The listing builds one solid part. Answer for the finished solid, in the listing's coordinates (mm). A direction names the side the tool comes from. Give positions to 0.01 mm unless a question says otherwise; leave off trailing zeros. Order: outer loops, then holes, each group sorted by start corner. A loop starts at its lowest first (then second) coordinate and runs counter-clockwise, first axis right, second up. Notation, with made-up numbers: (4, -3) - (42, -3) arc R13 ccw to (42, 19) - close; hole circle Ø1 at (86, -24). An arc over 180 degrees is marked (long way). Answer in a Markdown table with one row per item.
from build123d import *

# Parameters (mm, degrees)
SKETCH1_R                     = 9.5
SKETCH1_W                     = 7
SKETCH1_H                     = 1.9
BOSS_EXTRUDE1_DEPTH           = 50
SKETCH32_W                    = 32.172664372
SKETCH32_H                    = 50
SKETCH32_W_2                  = 30.763378825
BOSS_EXTRUDE4_DEPTH           = 3
SKETCH30_R                    = 1.675
SKETCH30_R_2                  = 1.25
CUT_EXTRUDE14_DEPTH           = 84.200435696
SKETCH31_R                    = 4
CUT_EXTRUDE15_DEPTH           = 2
CHAMFER1_SIZE                 = 1
SKETCH36_R                    = 2
CUT_EXTRUDE18_DEPTH           = 83.371475645
SKETCH37_R                    = 4
CUT_EXTRUDE19_DEPTH           = 2.8
SKETCH38_W                    = 7.194206864
SKETCH38_H                    = 7.080700956
BOSS_EXTRUDE6_DEPTH           = 6
BOSS_EXTRUDE6_DRAFT           = 20
BOSS_EXTRUDE6_PROFILE_2_DEPTH = 6
BOSS_EXTRUDE6_PROFILE_2_DRAFT = 20
FILLET2_R                     = 2
CHAMFER2_SIZE                 = 0.5
CUT_EXTRUDE20_START           = -10
SKETCH39_W                    = 33.713665857
SKETCH39_H                    = 35.884460507
CUT_EXTRUDE20_DEPTH           = 67.252868798
CUT_EXTRUDE21_DEPTH           = 83.371475645
CUT_EXTRUDE21_DEPTH_BACK      = 83.371475645
CHAMFER3_SIZE                 = 1
FILLET3_R                     = 2


with BuildPart() as part:
    # Sketch1 → Boss-Extrude1 (new body)
    with BuildSketch(Plane.XY):
        with BuildLine():
            Line((-34.408656248, 2.4), (34.408656248, 2.4))
            ThreePointArc((34.408656248, 2.4), (36.148562201, 2.95608362), (37.243446021, 4.418181818))
            ThreePointArc((37.243446021, 4.418181818), (52.24014746, 13.312841145), (63.5, 0))
            ThreePointArc((63.5, 0), (59.545941546, -9.545941546), (50, -13.5))
            ThreePointArc((50, -13.5), (42.170423209, -10.99762371), (37.243446021, -4.418181818))
            ThreePointArc((37.243446021, -4.418181818), (36.148562201, -2.95608362), (34.408656248, -2.4))
            Line((34.408656248, -2.4), (12.372954376, -2.4))
            ThreePointArc((12.372954376, -2.4), (10.729786704, -2.89001992), (9.623408959, -4.2))
            ThreePointArc((9.623408959, -4.2), (0, -10.5), (-9.623408959, -4.2))
            ThreePointArc((-9.623408959, -4.2), (-10.729786704, -2.89001992), (-12.372954376, -2.4))
            Line((-12.372954376, -2.4), (-34.408656248, -2.4))
            ThreePointArc((-34.408656248, -2.4), (-36.148562201, -2.95608362), (-37.243446021, -4.418181818))
            ThreePointArc((-37.243446021, -4.418181818), (-42.170423209, -10.99762371), (-50, -13.5))
            ThreePointArc((-50, -13.5), (-59.545941546, -9.545941546), (-63.5, 0))
            ThreePointArc((-63.5, 0), (-52.24014746, 13.312841145), (-37.243446021, 4.418181818))
            ThreePointArc((-37.243446021, 4.418181818), (-36.148562201, 2.95608362), (-34.408656248, 2.4))
        make_face()
        with Locations((50, 0)):
            Circle(SKETCH1_R, mode=Mode.SUBTRACT)
        with Locations(Location((-50, 0, 0), (0, 0, 180))):
            Circle(SKETCH1_R, mode=Mode.SUBTRACT)
        with Locations((0, -7.2)):
            Rectangle(SKETCH1_W, SKETCH1_H, mode=Mode.SUBTRACT)
    extrude(amount=BOSS_EXTRUDE1_DEPTH)

    # Sketch32 → Boss-Extrude4 (add)
    with BuildSketch(Plane.XZ.offset(2.4)):
        with Locations((-22.574766715, 25)):
            Rectangle(SKETCH32_W, SKETCH32_H)
        with Locations((23.370404996, 25)):
            Rectangle(SKETCH32_W_2, SKETCH32_H)
    extrude(amount=BOSS_EXTRUDE4_DEPTH)

    # Sketch30 → Cut-Extrude14 (cut, through all)
    with BuildSketch(Plane(origin=(0, -6.25, 0), x_dir=(1, 0, 0), z_dir=(0, 1, 0))):
        with Locations(Location((-0.160776584, -5, 0), (0, 0, 90))):
            Circle(SKETCH30_R)
        with Locations(Location((-0.160776584, -20, 0), (0, 0, 90))):
            Circle(SKETCH30_R)
        with Locations(Location((14.839223416, -12.5, 0), (0, 0, 90))):
            Circle(SKETCH30_R_2)
        with Locations(Location((-15.160776584, -12.5, 0), (0, 0, 90))):
            Circle(SKETCH30_R_2)
    extrude(amount=CUT_EXTRUDE14_DEPTH, mode=Mode.SUBTRACT)

    # Sketch31 → Cut-Extrude15 (cut)
    with BuildSketch(Plane(origin=(0, 2.4, 0), x_dir=(1, 0, 0), z_dir=(0, 1, 0))):
        with Locations(Location((-0.160776584, -5, 0), (0, 0, 270))):
            Circle(SKETCH31_R)
        with Locations(Location((-0.160776584, -20, 0), (0, 0, 270))):
            Circle(SKETCH31_R)
    extrude(amount=-CUT_EXTRUDE15_DEPTH, mode=Mode.SUBTRACT)

    # Chamfer1
    chamfer1_edges = [part.edges().sort_by_distance(p)[0] for p in [
        (0, -6.25, 0),
        (0, -6.25, 50),
    ]]
    chamfer(chamfer1_edges, length=CHAMFER1_SIZE)

    # Sketch36 → Cut-Extrude18 (cut, through all)
    with BuildSketch(Plane(origin=(0, 2.4, 0), x_dir=(1, 0, 0), z_dir=(0, 1, 0))):
        with Locations(Location((30, -10, 0), (0, 0, 270))):
            Circle(SKETCH36_R)
        with Locations(Location((-30, -10, 0), (0, 0, 270))):
            Circle(SKETCH36_R)
    extrude(amount=-CUT_EXTRUDE18_DEPTH, mode=Mode.SUBTRACT)

    # Sketch37 → Cut-Extrude19 (cut)
    with BuildSketch(Plane.XZ.offset(5.4)):
        with Locations((30, 10)):
            Circle(SKETCH37_R)
        with Locations((-30, 10)):
            Circle(SKETCH37_R)
    extrude(amount=-CUT_EXTRUDE19_DEPTH, mode=Mode.SUBTRACT)


with BuildPart() as boss_extrude6_tool:
    # Sketch38 → Boss-Extrude6 (with draft: the straight prism first)
    with BuildSketch(Plane(origin=(0, 2.4, 0), x_dir=(1, 0, 0), z_dir=(0, 0, 1))):
        with Locations((18.597103432, 0)):
            Rectangle(SKETCH38_W, SKETCH38_H)
    extrude(amount=BOSS_EXTRUDE6_DEPTH)
    # Boss-Extrude6: the draft: its side faces are tilted about the plane it starts from
    boss_extrude6_sides = [boss_extrude6_tool.faces().sort_by_distance(p)[0] for p in [
        (22.194206864, 2.4, 3),
        (18.597103432, 5.940350478, 3),
        (15, 2.4, 3),
        (18.597103432, -1.140350478, 3),
    ]]
    draft(boss_extrude6_sides, Plane(origin=(0, 2.4, 0), x_dir=(1, 0, 0), z_dir=(0, 0, 1)), BOSS_EXTRUDE6_DRAFT)


with BuildPart() as part_1:
    add(part.part)

    # Boss-Extrude6: add boss_extrude6_tool
    add(boss_extrude6_tool.part)


with BuildPart() as boss_extrude6_profile_2_tool:
    # Sketch38 → Boss-Extrude6 profile 2 (with draft: the straight prism first)
    with BuildSketch(Plane(origin=(0, 2.4, 0), x_dir=(1, 0, 0), z_dir=(0, 0, 1))):
        with Locations((-18.597103432, 0)):
            Rectangle(SKETCH38_W, SKETCH38_H)
    extrude(amount=BOSS_EXTRUDE6_PROFILE_2_DEPTH)
    # Boss-Extrude6 profile 2: the draft: its side faces are tilted about the plane it starts from
    boss_extrude6_profile_2_sides = [boss_extrude6_profile_2_tool.faces().sort_by_distance(p)[0] for p in [
        (-15, 2.4, 3),
        (-18.597103432, 5.940350478, 3),
        (-22.194206864, 2.4, 3),
        (-18.597103432, -1.140350478, 3),
    ]]
    draft(boss_extrude6_profile_2_sides, Plane(origin=(0, 2.4, 0), x_dir=(1, 0, 0), z_dir=(0, 0, 1)), BOSS_EXTRUDE6_PROFILE_2_DRAFT)


with BuildPart() as part_2:
    add(part_1.part)

    # Boss-Extrude6 profile 2: add boss_extrude6_profile_2_tool
    add(boss_extrude6_profile_2_tool.part)

    # Fillet2
    # the kernel refuses this fillet: 2 mm, written as the material it takes off along each edge
    with BuildSketch(Plane(origin=(23.632882776, 7.37902639, -3.952729582), x_dir=(0.11068304606838114, -0.946188648339465, -0.30409916978933155), z_dir=(-0.32361557711818506, -0.3236155771181852, 0.8891264907159881))) as fillet2_piece_1_section:
        with BuildLine():
            CenterArc((FILLET2_R * 0.889126490716, -FILLET2_R), FILLET2_R, 90, 83.282286536)
            Line((-FILLET2_R * 0.104008041637, -FILLET2_R * 0.883022221559), (0, 0))
            Line((0, 0), (FILLET2_R * 0.889126490716, 0))
        make_face()
    fillet2_piece_1 = extrude(amount=15.6394611, mode=Mode.PRIVATE)
    fillet2_piece_1 = split(fillet2_piece_1, bisect_by=Plane(origin=(20.940546386, 2.4, 2.229867585), z_dir=(0, 1, 0)), keep=Keep.TOP, mode=Mode.PRIVATE)
    add(fillet2_piece_1, mode=Mode.SUBTRACT)
    with BuildSketch(Plane(origin=(13.561324088, 7.37902639, -3.952729582), x_dir=(0.9461886483394653, 0.1106830460683812, -0.30409916978933144), z_dir=(0.3236155771181851, -0.32361557711818495, 0.8891264907159883))) as fillet2_piece_2_section:
        with BuildLine():
            CenterArc((FILLET2_R * 0.889126490716, -FILLET2_R), FILLET2_R, 90, 83.282286536)
            Line((-FILLET2_R * 0.104008041637, -FILLET2_R * 0.883022221559), (0, 0))
            Line((0, 0), (FILLET2_R * 0.889126490716, 0))
        make_face()
    fillet2_piece_2 = extrude(amount=15.6394611, mode=Mode.PRIVATE)
    fillet2_piece_2 = split(fillet2_piece_2, bisect_by=Plane(origin=(16.253660478, 2.4, 2.229867585), z_dir=(0, 1, 0)), keep=Keep.TOP, mode=Mode.PRIVATE)
    add(fillet2_piece_2, mode=Mode.SUBTRACT)
    with BuildSketch(Plane(origin=(-23.632882776, 7.37902639, -3.952729582), x_dir=(-0.11068304606838135, -0.9461886483394651, -0.3040991697893313), z_dir=(0.32361557711818506, -0.3236155771181851, 0.8891264907159881))) as fillet2_piece_3_section:
        with BuildLine():
            CenterArc((FILLET2_R * 0.889126490716, FILLET2_R), FILLET2_R, 186.717713464, 83.282286536)
            Line((-FILLET2_R * 0.104008041637, FILLET2_R * 0.883022221559), (0, 0))
            Line((0, 0), (FILLET2_R * 0.889126490716, 0))
        make_face()
    fillet2_piece_3 = extrude(amount=15.6394611, mode=Mode.PRIVATE)
    fillet2_piece_3 = split(fillet2_piece_3, bisect_by=Plane(origin=(-20.940546386, 2.4, 2.229867585), z_dir=(0, 1, 0)), keep=Keep.TOP, mode=Mode.PRIVATE)
    add(fillet2_piece_3, mode=Mode.SUBTRACT)
    with BuildSketch(Plane(origin=(-13.561324088, 7.37902639, -3.952729582), x_dir=(0.11068304606838107, -0.9461886483394651, -0.3040991697893313), z_dir=(-0.32361557711818506, -0.323615577118185, 0.8891264907159881))) as fillet2_piece_4_section:
        with BuildLine():
            CenterArc((FILLET2_R * 0.889126490716, -FILLET2_R), FILLET2_R, 90, 83.282286536)
            Line((-FILLET2_R * 0.104008041637, -FILLET2_R * 0.883022221559), (0, 0))
            Line((0, 0), (FILLET2_R * 0.889126490716, 0))
        make_face()
    fillet2_piece_4 = extrude(amount=15.6394611, mode=Mode.PRIVATE)
    fillet2_piece_4 = split(fillet2_piece_4, bisect_by=Plane(origin=(-16.253660478, 2.4, 2.229867585), z_dir=(0, 1, 0)), keep=Keep.TOP, mode=Mode.PRIVATE)
    add(fillet2_piece_4, mode=Mode.SUBTRACT)

    # Chamfer2
    chamfer2_edges = [part_2.edges().sort_by_distance(p)[0] for p in [
        (30, 2.4, 8),
        (-30, 2.4, 8),
    ]]
    chamfer(chamfer2_edges, length=CHAMFER2_SIZE)

    # Sketch39 → Cut-Extrude20 (cut, through all)
    with BuildSketch(Plane(origin=(0, 0, 10), x_dir=(-1, 0, 0), z_dir=(0, 0, -1)).offset(CUT_EXTRUDE20_START)):
        with Locations((50.736194558, -0.327009614)):
            Rectangle(SKETCH39_W, SKETCH39_H)
    extrude(amount=-CUT_EXTRUDE20_DEPTH, mode=Mode.SUBTRACT)

    # Sketch40 → Cut-Extrude21 (cut, two sides: drawn at the far end of the back side and taken through both)
    with BuildSketch(Plane(origin=(0, 2.4, 0), x_dir=(1, 0, 0), z_dir=(0, 1, 0)).offset(-CUT_EXTRUDE21_DEPTH_BACK)):
        Polygon((-33.879361629, -20), (95.398235412, -76.00132788), (-43.756067754, -79.660476008), align=None)
    extrude(amount=CUT_EXTRUDE21_DEPTH + CUT_EXTRUDE21_DEPTH_BACK, mode=Mode.SUBTRACT)

    # Chamfer3
    chamfer3_edges = [part_2.edges().sort_by_distance(p)[0] for p in [
        (-40.5, 0, 20),
        (0, -6.25, 34.676086827),
        (40.5, 0, 0),
        (40.5, 0, 50),
        (-40.5, 0, 0),
    ]]
    chamfer(chamfer3_edges, length=CHAMFER3_SIZE)

    # Fillet3
    fillet3_edges = [part_2.edges().sort_by_distance(p)[0] for p in [
        (-33.879361629, -1.5, 20),
        (35.374851763, -1.42007625, 50),
        (-37.627045624, -5.4, 10),
        (37.627045624, -5.4, 25),
    ]]
    fillet(fillet3_edges, radius=FILLET3_R)


solid = part_2.part
Item 1: Find section B-B on z = 42. Write down the section's boundary in (x, y), then the cut area to 3 significant figures.
Answer block:
| item | result |
|---|---|
| outline | (16.91, -5.4) - (36.38, -5.4) arc R2 cw to (38.14, -6.45) arc R13.5 ccw (long way) to (37.24, 4.42) arc R3 cw to (34.41, 2.4) - (16.91, 2.4) - close; hole circle Ø19 at (50, 0) |
| area | 445 mm² |
Item 2: Each of these flat-tipped pins is pushed along its axis until it touches: P1, Ø3.5, axis at x = -30, z = 10, coming from the -Y side; P2, Ø1, axis at x = 19, y = 3, coming from the +Z side; P3, Ø2, axis at x = -0.16, z = 5, coming from the -Y side; P4, Ø5, axis at x = -13.5, z = 29, coming from the -Y side. Where does it stop, or does it pass through?
Answer block:
| item | result |
|---|---|
| P1 | through |
| P2 | z = 6 |
| P3 | y = -10.5 |
| P4 | y = -5.4 |
Item 3: Determine the mould class of faces 1 (the face through (-30.521, -4.02, 13.966)), 2 (the face through (36.127, 2.941, 24.65)), 3 (the face through (0, -8.15, 18)) for opening direction Y: pulls with the +Y half, pulls with the -Y half, needs draft (parallel to the pull), parting line crosses it, or undercut.
Answer block:
| item | result |
|---|---|
| face 1 | needs draft |
| face 2 | pulls with the +Y half |
| face 3 | undercut |
Item 4: Consider line 1 (X direction, y = -2.25, z = 12.5); line 2 (X direction, y = 0.5, z = 12.5); line 3 (Y direction, x = -50, z = 6). Determine where each line is inside the solid, lowest interval first.
Answer block:
| item | result |
|---|---|
| line 1 | -63.31 to -59.23, -40.77 to -16.41, -13.91 to 13.59, 16.09 to 40.77, 59.23 to 63.31 |
| line 2 | -63.49 to -59.49, -40.51 to -16.41, -13.91 to 13.59, 16.09 to 40.51, 59.49 to 63.49 |
| line 3 | -13.5 to -9.5, 9.5 to 13.5 |
Item 5: Find section A-A on y = 12. Write down the section's boundary in (x, z), then the cut area to 3 significant figures.
Answer block:
| item | result |
|---|---|
| outline | (-56.18, 0) - (-43.82, 0) - (-43.82, 20) - (-56.18, 20) - close; (43.82, 0) - (56.18, 0) - (56.18, 50) - (43.82, 50) - close |
| area | 866 mm² |
Item 6: Which of the six approach directions +Z, -Z, +X, -X, +Y, -Y give full straight-line access (tool end or side, diameter ignored) to faces 4 (the face through (-29, -2.6, 12)), 5 (the face through (-20.55, 4.33, 2.99)), 6 (the face through (-40, -4, 20)), 7 (the face through (0.055, -5.757, 34.147))?
Answer block:
| item | result |
|---|---|
| face 4 | -Y |
| face 5 | +Z, +Y |
| face 6 | +Z, -X, +Y, -Y |
| face 7 | +Z |
